CAD build for the part. Positions are in the model's coordinates, mm. Coordinates: 2 decimals unless noted, no trailing zeros. Write each loop counter-clockwise with the first axis right and the second up, starting at its lowest first coordinate (ties: lowest second). Pieces come first, ordered by that corner, then holes. Notation, with made-up numbers: (86.25, 18) -> (109.25, 18) arc R25 ccw to (109.25, 52) -> close; hole circle Ø7 at (72.25, -21). An arc over 180 degrees is marked (long way). Answer as CSV lines item,"result".
```python
from build123d import *

# Parameters (mm, degrees)
F0_W     = 42.8625
F0_H     = 42.8625
F0_R     = 10.31875
F1_DEPTH = 21.336
F2_R     = 0.508


with BuildPart() as f1:
    # F0 (on Top) → F1 (new body)
    with BuildSketch(Plane.XY):
        with Locations((28.250322, -26.592983)):
            Rectangle(F0_W, F0_H)
        with Locations((28.250322, -26.592983)):
            Circle(F0_R, mode=Mode.SUBTRACT)
    extrude(amount=F1_DEPTH)

    # F2
    f2_edges = [f1.edges().sort_by_distance(p)[0] for p in [
        (28.250322, -5.161733, 0),
        (6.819072, -5.161733, 10.668),
        (28.250322, -5.161733, 21.336),
        (49.681572, -5.161733, 10.668),
        (6.819072, -26.592983, 0),
        (28.250322, -48.024233, 0),
        (49.681572, -26.592983, 0),
        (17.931572, -26.592983, 0),
        (49.681572, -48.024233, 10.668),
        (49.681572, -26.592983, 21.336),
        (6.819072, -26.592983, 21.336),
        (28.250322, -48.024233, 21.336),
        (17.931572, -26.592983, 21.336),
        (6.819072, -48.024233, 10.668),
    ]]
    fillet(f2_edges, radius=F2_R)


solid = f1.part
```
Item 1: Wall check: line 1 (X direction, y = -27, z = 7.5); line 2 (X direction, y = -27.5, z = 20.25); line 3 (Y direction, x = 19, z = 2.25). Give the ranges that are in metal, low to high. Write a range as from..to.
Answer below:
line 1,"x = 6.82..17.94, 38.56..49.68"
line 2,"x = 6.82..17.97, 38.53..49.68"
line 3,"y = -48.02..-31.17, -22.02..-5.16"
Item 2: Flat gauge pin, fed straight in: pin 1 (10 mm diameter, centred on x = 15, y = -21.5, fed in from -Z). Where does the tip first touch, or does it go through?
Answer below:
pin 1,"stops at z = 0"
Item 3: Saw through at A-A on z = 15. Give the cut face in (x, y), and give its area (3 significant figures).
Answer below:
outline,"(6.82, -47.52) arc R0.51 ccw to (7.33, -48.02) -> (49.17, -48.02) arc R0.51 ccw to (49.68, -47.52) -> (49.68, -5.67) arc R0.51 ccw to (49.17, -5.16) -> (7.33, -5.16) arc R0.51 ccw to (6.82, -5.67) -> close; hole circle Ø20.64 at (28.25, -26.59)"
area,"1,500 mm2"
Item 4: Two-plate mould, pull along Y, no slides. Class faces 1 (the cylindrical face through (38.09, -23.49, 10.53)), 2 (the flat face through (28, -48.024, 11)), 3 (the flat face through (6.819, -27, 11)), 4 (the flat face through (28, -5.162, 11)): pulls with the +Y half, pulls with the -Y half, needs draft (parallel to the pull), parting line crosses it, or undercut.
Answer below:
face 1,"undercut"
face 2,"pulls with the -Y half"
face 3,"needs draft"
face 4,"pulls with the +Y half"
